```python
from build123d import *

# Parameters (mm, degrees)
SKETCH1_W            = 70
SKETCH1_H            = 48
BOSS_EXTRUDE1_DEPTH  = 1.5
BOSS_EXTRUDE6_DEPTH  = 70
BOSS_EXTRUDE7_DEPTH  = 1.5
BOSS_EXTRUDE8_DEPTH  = 1.5
SKETCH9_R            = 5
BOSS_EXTRUDE9_DEPTH  = 10
SKETCH10_R           = 2.8
CUT_EXTRUDE1_DEPTH   = 8
SKETCH11_W           = 48
SKETCH11_H           = 36
CUT_EXTRUDE2_DEPTH   = 1.6
BOSS_EXTRUDE10_REACH = 74.403
SKETCH12_W           = 2.5
SKETCH12_H           = 48


with BuildPart() as part:
    # Sketch1 → Boss-Extrude1 (new body)
    with BuildSketch(Plane(origin=(0, 0, 0), x_dir=(1, 0, 0), z_dir=(0, 1, 0))):
        with Locations((-11.991596639, -2.521008403)):
            Rectangle(SKETCH1_W, SKETCH1_H)
    extrude(amount=BOSS_EXTRUDE1_DEPTH)

    # Sketch6 → Boss-Extrude6 (add)
    with BuildSketch(Plane(origin=(23.008403361, 0, 0), x_dir=(0, 0, -1), z_dir=(1, 0, 0))):
        Polygon((18.978991597, 1.5), (21.478991597, 1.5), (21.478991597, 8), (-26.521008403, 48.276782297), (-26.521008403, 45.013264073), (-24.021008403, 42.915514995), (18.978991597, 6.834230855), align=None)
    extrude(amount=-BOSS_EXTRUDE6_DEPTH)

    # Sketch7 → Boss-Extrude7 (add)
    with BuildSketch(Plane(origin=(23.008403361, 0, 0), x_dir=(0, 0, -1), z_dir=(1, 0, 0))):
        Polygon((-26.521008403, 1.5), (18.978991597, 1.5), (18.978991597, 6.834230855), (-26.521008403, 45.013264073), align=None)
    extrude(amount=-BOSS_EXTRUDE7_DEPTH)

    # Sketch8 → Boss-Extrude8 (add)
    with BuildSketch(Plane.ZY.offset(46.991596639)):
        Polygon((-18.978991597, 6.834230855), (26.521008403, 45.013264073), (26.521008403, 1.5), (-18.978991597, 1.5), align=None)
    extrude(amount=-BOSS_EXTRUDE8_DEPTH)

    # Sketch9 → Boss-Extrude9 (add)
    with BuildSketch(Plane.XZ):
        with Locations((17.008403361, -15.478991597)):
            Circle(SKETCH9_R)
        with Locations((-40.991596639, -15.478991597)):
            Circle(SKETCH9_R)
        with Locations((-40.991596639, 20.521008403)):
            Circle(SKETCH9_R)
        with Locations((17.008403361, 20.521008403)):
            Circle(SKETCH9_R)
    extrude(amount=-BOSS_EXTRUDE9_DEPTH)

    # Sketch10 → Cut-Extrude1 (cut)
    with BuildSketch(Plane.XZ):
        with Locations(Location((17.008403361, -15.478991597, 0), (0, 0, 270))):
            Circle(SKETCH10_R)
        with Locations(Location((-40.991596639, -15.478991597, 0), (0, 0, 270))):
            Circle(SKETCH10_R)
        with Locations(Location((-40.991596639, 20.521008403, 0), (0, 0, 270))):
            Circle(SKETCH10_R)
        with Locations(Location((17.008403361, 20.521008403, 0), (0, 0, 270))):
            Circle(SKETCH10_R)
    extrude(amount=-CUT_EXTRUDE1_DEPTH, mode=Mode.SUBTRACT)

    # Sketch11 → Cut-Extrude2 (cut)
    with BuildSketch(Plane.XZ):
        with Locations((-11.991596639, 2.521008403)):
            Rectangle(SKETCH11_W, SKETCH11_H)
    extrude(amount=-CUT_EXTRUDE2_DEPTH, mode=Mode.SUBTRACT)

    # Boss-Extrude10: up to this plane
    boss_extrude10_end = Plane(origin=(-46.991596639, 13.355820328, -11.206863912), z_dir=(0, 0.7660444431189827, -0.6427876096865339))
    # Sketch12 → Boss-Extrude10 (add, up to the surface)
    with BuildSketch(Plane.XZ, mode=Mode.PRIVATE) as boss_extrude10_sk1:
        with Locations((-11.991596639, 2.521008403)):
            Rectangle(SKETCH12_W, SKETCH12_H)
    boss_extrude10_tool1 = split(extrude(boss_extrude10_sk1.sketch, amount=-BOSS_EXTRUDE10_REACH, mode=Mode.PRIVATE), bisect_by=boss_extrude10_end, keep=Keep.BOTH, mode=Mode.PRIVATE)
    add(boss_extrude10_tool1.solids().sort_by_distance((-11.991597, 0, 2.521008))[0])


solid = part.part
```
Work out the finished part from the listing and answer in its coordinate system (mm). A direction names the side the tool comes from. Give positions to 0.01 mm unless a question says otherwise; leave off trailing zeros. Write each loop counter-clockwise with the first axis right and the second up, starting at its lowest first coordinate (ties: lowest second). Pieces come first, ordered by that corner, then holes.
(1) The part is cut by section D-D on y = 44. Write down the section's boundary in (x, z).
Final values:
outline: (-46.99, 21.42) - (23.01, 21.42) - (23.01, 26.52) - (21.51, 26.52) - (21.51, 25.31) - (-10.74, 25.31) - (-10.74, 26.52) - (-13.24, 26.52) - (-13.24, 25.31) - (-45.49, 25.31) - (-45.49, 26.52) - (-46.99, 26.52) - close
(2) The part is cut by section A-A on x = -35. Write down the section's boundary in (y, z).
Final values:
outline: (0, -21.48) - (8, -21.48) - (48.28, 26.52) - (45.01, 26.52) - (6.83, -18.98) - (1.5, -18.98) - (1.5, -15.48) - (0, -15.48) - close; (0, 20.52) - (1.5, 20.52) - (1.5, 26.52) - (0, 26.52) - close
(3) The part is cut by section C-C on y = 13. Write down the section's boundary in (x, z).
Final values:
outline: (-46.99, -15.52) - (23.01, -15.52) - (23.01, 26.52) - (21.51, 26.52) - (21.51, -11.63) - (-10.74, -11.63) - (-10.74, 26.52) - (-13.24, 26.52) - (-13.24, -11.63) - (-45.49, -11.63) - (-45.49, 26.52) - (-46.99, 26.52) - close
(4) Which of the six approach directions +Z, -Z, +X, -X, +Y, -Y give full straight-line access (tool end or side, diameter ignored) to faces 5 (the flat face through (2, 1.5, 23)), 6 (the flat face through (17, 8, -15)), 7 (the flat face through (-45.492, 19, 11))?
Final values:
face 5: +Z
face 6: -Y
face 7: none
(5) Straight lines are drawn through the part: line 1 (X direction, y = 33, z = 21.5); line 2 (Z direction, x = -25, y = 5.5); line 3 (Y direction, x = 14.5, z = 10). For each, find the intervals that lie inside material, in ascending order.
Final values:
line 1: x = -46.99 to -45.49, -13.24 to -10.74, 21.51 to 23.01
line 2: z = -21.48 to -18.98
line 3: y = 0 to 1.5, 31.15 to 34.41
(6) Flat-ended cylindrical pins translate along their axes: pin 1 Ø4 at (x, z) = (-30.5, 20) entering from -Y; pin 2 Ø1.1 at (x, z) = (-2, -16.5) entering from +Y; pin 3 Ø1.1 at (x, z) = (-24, -18) entering from +Y; pin 4 Ø1.7 at (x, z) = (-40.5, 19.5) entering from -Y. Find the tip coordinate at first contact, or state that the pin passes through.
Final values:
pin 1: stops at y = 0
pin 2: stops at y = 12.64
pin 3: stops at y = 11.38
pin 4: stops at y = 8
(7) The part is cut by section B-B on z = -4. Write down the section's boundary in (x, y), plus the area to 3 significant figures.
Final values:
outline: (-46.99, 0) - (-35.99, 0) - (-35.99, 1.5) - (-45.49, 1.5) - (-45.49, 19.4) - (-13.24, 19.4) - (-13.24, 0) - (-10.74, 0) - (-10.74, 19.4) - (21.51, 19.4) - (21.51, 1.5) - (12.01, 1.5) - (12.01, 0) - (23.01, 0) - (23.01, 22.67) - (-46.99, 22.67) - close
area: 364 mm2
(8) The mould has two halves that part along X. Classify faces 1 (the flat face through (-12, 0, 3)), 2 (the cylindrical face through (-38.02, 5.69, -11.46)), 3 (the cylindrical face through (-42.7, 3.94, 22.74)), 4 (the flat face through (-46.992, 19, 8)): pulls with the +X half, pulls with the -X half, needs draft (parallel to the pull), parting line crosses it, or undercut.
Final values:
face 1: needs draft
face 2: undercut
face 3: undercut
face 4: pulls with the -X half
